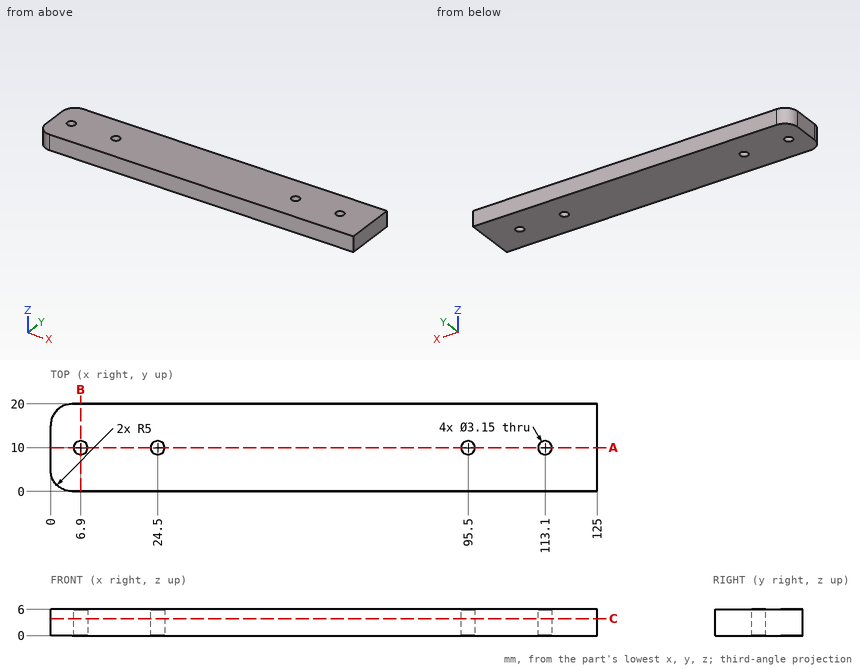
Source: three-view drawing plus pictorial views. Frame: mm from the lowest corner of the part. Give positions to 0.01 mm unless a question says otherwise; leave off trailing zeros. Order: outer loops, then holes, each group sorted by start corner. A loop starts at its lowest first (then second) coordinate and runs counter-clockwise, first axis right, second up. Notation, with made-up numbers: (-10, -24) - (41, -24) arc R17 cw to (41, -10) - close; hole circle Ø3 at (64, 77). An arc over 180 degrees is marked (long way). Answer as a JSON object with one key per item and string values. Group by question number.
Q1. Cut plane A-A, the plane y = 10. Output: boundary loops of the cut face in (x, z) (3 decimals).
Q2. Cut plane B-B, the plane x = 6.9. Output: boundary loops of the cut face in (y, z) (3 decimals), then the cut area to 3 significant figures.
Q3. Cut plane C-C, the plane z = 3.9. Output: boundary loops of the cut face in (x, y) (3 decimals).
Q4. First-contact query: pin 1 Ø1 at (y, z) = (4, 5) entering from -X; pin 2 Ø2.5 at (x, y) = (24.5, 10) entering from -Z; pin 3 Ø5 at (x, y) = (95.5, 10) entering from +Z. Flat tips, straight axial feed; report the tip coordinate or a pass-through.
Q5. Line query: probe 1 along Y at (x, z) = (6.9, 2.4) (3 decimals); probe 2 along X at (y, z) = (11, 1.3); probe 3 along X at (y, z) = (9.5, 2). Output: solid intervals per line, ascending.
Results:
{
 "1": {"outline": "(0, 0) - (5.325, 0) - (5.325, 6) - (0, 6) - close; (8.475, 0) - (22.925, 0) - (22.925, 6) - (8.475, 6) - close; (26.075, 0) - (93.925, 0) - (93.925, 6) - (26.075, 6) - close; (97.075, 0) - (111.525, 0) - (111.525, 6) - (97.075, 6) - close; (114.675, 0) - (125, 0) - (125, 6) - (114.675, 6) - close"},
 "2": {"outline": "(0, 0) - (8.425, 0) - (8.425, 6) - (0, 6) - close; (11.575, 0) - (20, 0) - (20, 6) - (11.575, 6) - close", "area": "101 mm^2"},
 "3": {"outline": "(0, 5) arc R5 ccw to (5, 0) - (125, 0) - (125, 20) - (5, 20) arc R5 ccw to (0, 15) - close; hole circle Ø3.15 at (6.9, 10); hole circle Ø3.15 at (24.5, 10); hole circle Ø3.15 at (95.5, 10); hole circle Ø3.15 at (113.1, 10)"},
 "4": {"pin 1": "x = 0.03", "pin 2": "through", "pin 3": "z = 6"},
 "5": {"probe 1": "0 to 8.425, 11.575 to 20", "probe 2": "0 to 5.68, 8.12 to 23.28, 25.72 to 94.28, 96.72 to 111.88, 114.32 to 125", "probe 3": "0 to 5.41, 8.39 to 23.01, 25.99 to 94.01, 96.99 to 111.61, 114.59 to 125"}
}
